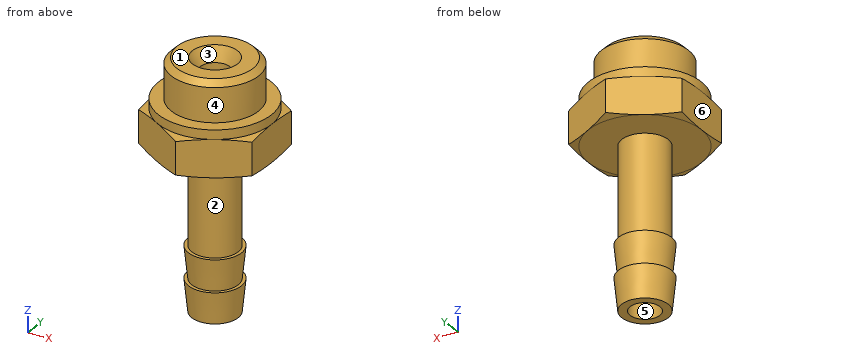
Autodesk Inventor part; units mm, degrees
ref_plane "ANBAU_STD_XY" through (0, 0, -6) normal (0, 0, -1) x (1, 0, 0)
ref_plane "ANBAU_STD_YZ" through (0, 0, -6) normal (1, 0, 0) x (0, -1, 0)
ref_plane "ANBAU_STD_ZX" through (0, 0, -6) normal (0, -1, 0) x (0, 0, -1)
sketch "Skizze_1" plane through (0, 0, 0) normal (1, 0, 0) x (0, 1, 0)
  line L0 (0, -37.1) -> (0, 0)
  line L1 (0, 0) -> (5.7225, 0)
  line L2 (5.7225, 0) -> (6.5785, -0.856)
  line L3 (6.5785, -0.856) -> (6.5785, -6)
  line L4 (6.5785, -6) -> (8.5, -6)
  line L5 (8.5, -6) -> (8.5, -7.4)
  line L6 (8.5, -7.4) -> (10.2, -7.8555)
  line L7 (10.2, -7.8555) -> (10.2, -12.5445)
  line L8 (10.2, -12.5445) -> (8.5, -13)
  line L9 (8.5, -13) -> (3.5, -13)
  line L10 (3.5, -13) -> (3.5, -27.46)
  line L11 (3.5, -27.46) -> (4, -27.46)
  line L12 (4, -27.46) -> (3.5, -32.28)
  line L13 (3.5, -32.28) -> (4, -32.28)
  line L14 (4, -32.28) -> (3.5, -37.1)
  line L15 (3.5, -37.1) -> (0, -37.1)
  line L16 (0, -37.1) -> (0, 0)
revolve "Revolution1" add sketch "Skizze_1" angle 360 about axis through (0, 0, -37.1) along (0, 0, -1)
thread "Thread1"
sketch "Sketch2" plane through (0, 0, 0) normal (0, 0, 1) x (1, 0, 0)
  point P0 (0, 0)
hole "Hole1" at (0, 0, 0) direction (0, 0, -1) diameter 4.5 depth 37.1 countersink diameter 6.8094 countersink angle 60
sketch "Skizze_3" plane through (0, 0, 0) normal (0, 0, 1) x (1, 0, 0)
  line L0 (-17, -17) -> (17, -17)
  line L1 (17, -17) -> (17, 17)
  line L2 (17, 17) -> (-17, 17)
  line L3 (-17, 17) -> (-17, -17)
  line L4 (-8.5, -4.9075) -> (0, -9.815)
  line L5 (0, -9.815) -> (8.5, -4.9075)
  line L6 (8.5, -4.9075) -> (8.5, 4.9075)
  line L7 (8.5, 4.9075) -> (0, 9.815)
  line L8 (0, 9.815) -> (-8.5, 4.9075)
  line L9 (-8.5, 4.9075) -> (-8.5, -4.9075)
extrude "Extrusion1" cut sketch "Skizze_3" against normal blind 13
ref_plane "ANBAU_STD_XY" through (0, 0, -6) normal (0, 0, -1) x (1, 0, 0)
ref_plane "ANBAU_STD_YZ" through (0, 0, -6) normal (1, 0, 0) x (0, -1, 0)
ref_plane "ANBAU_STD_ZX" through (0, 0, -6) normal (0, -1, 0) x (0, 0, -1)
properties part number "15631 N-1/4-P-6-MS"
Input: part model. Units: mm. Frame: model coordinates. Face numbers are marked on the shaded views. A direction names the side the tool comes from. Coordinates: 2 decimals unless noted, no trailing zeros. Write each loop counter-clockwise with the first axis right and the second up, starting at its lowest first coordinate (ties: lowest second). Pieces come first, ordered by that corner, then holes. Notation, with made-up numbers: (-40, 7.25) -> (-1, 7.25) arc R23 cw to (-1, 25.25) -> close; hole circle Ø6 at (-38.75, -22.5). An arc over 180 degrees is marked (long way). Write each question's results on one line, items separated by ' | '.
Item 1: Pin query (flat end, axial travel): pin 1 Ø1 at (x, y) = (-4, 3.5) entering from -Z. Return the tip coordinate at first contact, or that it passes through.
Conclusion:
pin 1: stops at z = -13
Item 2: Set-up query: the marked faces 1 and 2. Return all of +Z, -Z, +X, -X, +Y, -Y with unobstructed straight access to the full face (end or side cutting, diameter ignored); none if empty.
Conclusion:
face 1: +Z, +X, -X, +Y, -Y | face 2: none
Item 3: Section query B-B on z = -15.5. Return loops of the section in (x, y).
Conclusion:
outline: circle Ø7 at (0, 0); hole circle Ø4.5 at (0, 0)
Item 4: Mould query, pull axis X, two halves, no side actions, for the marked faces 3, 4, 5 and 6. Classes: +X half, -X half, draft (parallel to the pull), parting line (faces both ways), or undercut.
Conclusion:
face 3: undercut | face 4: parting line | face 5: undercut | face 6: -X half
Item 5: Material intervals for probe 1 along X at (y, z) = (0, -10); probe 2 along Y at (x, z) = (0, -27.5); probe 3 along X at (y, z) = (0, -24), sorted ascending.
Conclusion:
probe 1: x = -8.5 to -2.25, 2.25 to 8.5 | probe 2: y = -4 to -2.25, 2.25 to 4 | probe 3: x = -3.5 to -2.25, 2.25 to 3.5
